Design review of the part built by this model. Coordinates are the model's own, in mm. A direction names the side the tool comes from. Coordinates: 2 decimals unless noted, no trailing zeros. Loops run counter-clockwise (first coordinate to the right, second up) from the corner with the lowest first, then second, coordinate; pieces in that order, holes last. Notation, with made-up numbers: (19, 83.5) -> (59, 83.5) arc R25 cw to (59, 98.5) -> close; hole circle Ø3 at (6.25, -18.5). An arc over 180 degrees is marked (long way). Answer in a Markdown table with one row per item.
Autodesk Inventor part; units mm, degrees
ref_plane "YZ Plane" through (0, 0, 0) normal (1, 0, 0) x (0, 1, 0)
ref_plane "XZ Plane" through (0, 0, 0) normal (0, 1, 0) x (-1, 0, 0)
ref_plane "XY Plane" through (0, 0, 0) normal (0, 0, 1) x (1, 0, 0)
sketch "Эскиз1" plane through (0, 0, 0) normal (0, 0, 1) x (1, 0, 0)
  circle A0 centre (0, 0) radius 9.5
  circle A1 centre (0, 0) radius 12.5
  circle A2 centre (0, 0) radius 19.6
  circle A3 centre (-19.6, 0) radius 2.1
  circle A4 centre (19.6, 0) radius 2.1
  line L0 (-21.7, 0) -> (21.7, 0)
  line L1 (-25.6, 6) -> (25.6, 6)
  line L2 (-25.6, -6) -> (25.6, -6)
  line L3 (-25.6, 6) -> (-25.6, -6)
  line L4 (0, 0) -> (0, 6)
  line L5 (25.6, 6) -> (25.6, -6)
  point P0 (10.9659, -6)
  point P1 (10.9659, 6)
  point P2 (-10.9659, 6)
  point P3 (-10.9659, -6)
  dimension "d3" = 4.2
  dimension "d4" = 4.2
  dimension "d0" = 19
  dimension "d1" = 25
  dimension "d2" = 39.2
  dimension "d5" = 6
  dimension "d6" = 6
  dimension "d7" = 6
extrude "Выдавливание1" add sketch "Эскиз1" along normal blind 3 contours L0 A1 L2 A0 | A0 L1 A1 L0 | A0 L1 A1 | L2 A1 A0 | L0 A4 A2 L2 A1 | A1 L1 A2 A4 L0 | A0 L0 A1 L1 | L2 A1 L0 A0 | A1 L0 A3 A2 L1 | L1 L5 L2 A2 A4 | L2 A2 A3 L0 A1 | A2 A3 L2 L3 L1
sketch "Эскиз2" plane through (0, 0, 0) normal (0, 0, -1) x (-1, 0, 0)
  line L0 (-25.6, -6) -> (-25.6, 6)
  line L1 (-10.9659, -6) -> (-25.6, -6)
  arc A0 (-10.9659, -6) -> (10.9659, -6) centre (0, 0) ccw
  line L2 (25.6, -6) -> (10.9659, -6)
  line L3 (25.6, 6) -> (25.6, -6)
  line L4 (10.9659, 6) -> (25.6, 6)
  arc A1 (10.9659, 6) -> (-10.9659, 6) centre (0, 0) ccw
  line L5 (-25.6, 6) -> (-10.9659, 6)
  circle A2 centre (-19.6, 0) radius 2.1
  circle A3 centre (19.6, 0) radius 2.1
  circle A4 centre (0, 0) radius 9.5
  circle A5 centre (0, 0) radius 12.5
  point P0 (-10.9659, 6)
extrude "Выдавливание2" add sketch "Эскиз2" along normal blind 4 contours A5 A1 A0
sketch "Эскиз3" plane through (0, 0, -4) normal (0, 0, -1) x (-1, 0, 0)
  circle A0 centre (0, 0) radius 12.5
  circle A1 centre (0, 0) radius 9.5
  circle A2 centre (0, 0) radius 3.1
  dimension "d12" = 6.2
extrude "Выдавливание3" add sketch "Эскиз3" along normal blind 3.2 contours A0 | A1
fillet "Сопряжение1" radius 5 8 edges at (-25.6, 6, 1.5) (-25.6, -6, 1.5) (25.6, 6, 1.5) (25.6, -6, 1.5) (10.9659, -6, 1.5) (10.9659, 6, 1.5) (-10.9659, 6, 1.5) (-10.9659, -6, 1.5)
properties part number "для подшипника 25-26"
(1) Draft analysis for pull direction X (two halves, no side actions). For faces 1 (the cylindrical face through (0.2, 12.5, -2)), 2 (the cylindrical face through (24.17, 4.5, 1.52)), 3 (the flat face through (0, -4, -4)), 4 (the flat face through (-17, -6, 1)), state which applies: pulls with the +X half, pulls with the -X half, needs draft (parallel to the pull), parting line crosses it, or undercut.
Evaluation:
| item | result |
|---|---|
| face 1 | parting line crosses it |
| face 2 | pulls with the +X half |
| face 3 | undercut |
| face 4 | needs draft |
(2) Take a section at C-C on z = -5.5. Give the boundary of the cut face in (x, y), and give its area (3 significant figures).
Evaluation:
| item | result |
|---|---|
| outline | circle Ø25 at (0, 0); hole circle Ø6.2 at (0, 0) |
| area | 461 mm² |
(3) Take a section at A-A on x = 19.6. Give the boundary of the cut face in (y, z), and give its area (3 significant figures).
Evaluation:
| item | result |
|---|---|
| outline | (-6, 0) -> (-2.1, 0) -> (-2.1, 3) -> (-6, 3) -> close; (2.1, 0) -> (6, 0) -> (6, 3) -> (2.1, 3) -> close |
| area | 23.4 mm² |
(4) Take a section at D-D on y = 10.25. Give the boundary of the cut face in (x, z), and give its area (3 significant figures).
Evaluation:
| item | result |
|---|---|
| outline | (-7.15, -7.2) -> (7.15, -7.2) -> (7.15, 0) -> (7.15, 3) -> (-7.15, 3) -> (-7.15, 0) -> close |
| area | 146 mm² |
(5) Take a section at B-B on x = 0. Give the boundary of the cut face in (y, z).
Evaluation:
| item | result |
|---|---|
| outline | (-12.5, -7.2) -> (-3.1, -7.2) -> (-3.1, -4) -> (-9.5, -4) -> (-9.5, 3) -> (-12.5, 3) -> (-12.5, 0) -> close; (3.1, -7.2) -> (12.5, -7.2) -> (12.5, 0) -> (12.5, 3) -> (9.5, 3) -> (9.5, -4) -> (3.1, -4) -> close |
(6) Tool access review of faces 5 (the cylindrical face through (21.603, -0.631, 1.479)), 6 (the cylindrical face through (-0.2, -12.5, -2)), 7 (the flat face through (17, 6, 1)): name each direction out of +Z, -Z, +X, -X, +Y, -Y from which nothing blocks a thin tool from reaching the whole face with its end or side.
Evaluation:
| item | result |
|---|---|
| face 5 | +Z, -Z |
| face 6 | -Z, -Y |
| face 7 | +Z, -Z, +X, +Y |
(7) For pin 1 (4 mm diameter, centred on x = -20.5, y = 1.5, fed in from -Z); pin 2 (1.5 mm diameter, centred on x = 16, z = 1, fed in from +Y); pin 3 (9.5 mm diameter, centred on x = 4, y = 3, fed in from +Z); pin 4 (5.5 mm diameter, centred on x = 0, y = 0, fed in from +Z), all flat-tipped, find the tip position at first contact; note any pin that passes through.
Evaluation:
| item | result |
|---|---|
| pin 1 | stops at z = 0 |
| pin 2 | stops at y = 6 |
| pin 3 | stops at z = 3 |
| pin 4 | passes through |
(8) To check wall thickness, follow probe 1 along X at (y, z) = (0, 1.45); probe 2 along Y at (x, z) = (19.6, 1.35); probe 3 along Y at (x, z) = (-8.5, 2.75). State the ranges of each line that lie inside material, in increasing order.
Evaluation:
| item | result |
|---|---|
| probe 1 | x = -25.6 to -21.7, -17.5 to -9.5, 9.5 to 17.5, 21.7 to 25.6 |
| probe 2 | y = -6 to -2.1, 2.1 to 6 |
| probe 3 | y = -9.17 to -4.24, 4.24 to 9.17 |
